Verification items for this drawing (mm, ordinates from the low corner). Coordinates: 2 decimals unless noted, no trailing zeros. Write each loop counter-clockwise with the first axis right and the second up, starting at its lowest first coordinate (ties: lowest second). Pieces come first, ordered by that corner, then holes. Notation, with made-up numbers: M -7,-20.5 L 41,-20.5 A15 cw 41,4.5 Z; hole C 12.5,4.25 d2. An arc over 180 degrees is marked long. Put each result on its own line as item: value. Start each with the question number.
1) Cross-section at C-C on z = 237.5. Record the cut outline in (x, y).
2) Cross-section at A-A on x = 32.5. Record the cut outline in (y, z).
3) Cross-section at D-D on y = 150.5. Record the cut outline in (x, z).
4) Cross-section at B-B on y = 40.5. Record the cut outline in (x, z).
5) Gauge pin test, flat ends, axial feed: pin 1 (8 mm diameter, centred on y = 167.5, z = 715.5, fed in from +X); pin 2 (1.5 mm diameter, centred on y = 124.5, z = 723, fed in from -X). Record the tip position at first contact, or that the pin passes through.
6) Scan lines: line 1 along X through (y, z) = (156, 626); line 2 along Z through (x, y) = (48, 13.5); line 3 along Y through (x, z) = (32.5, 671). Record each from-to range of solid material in increasing order.
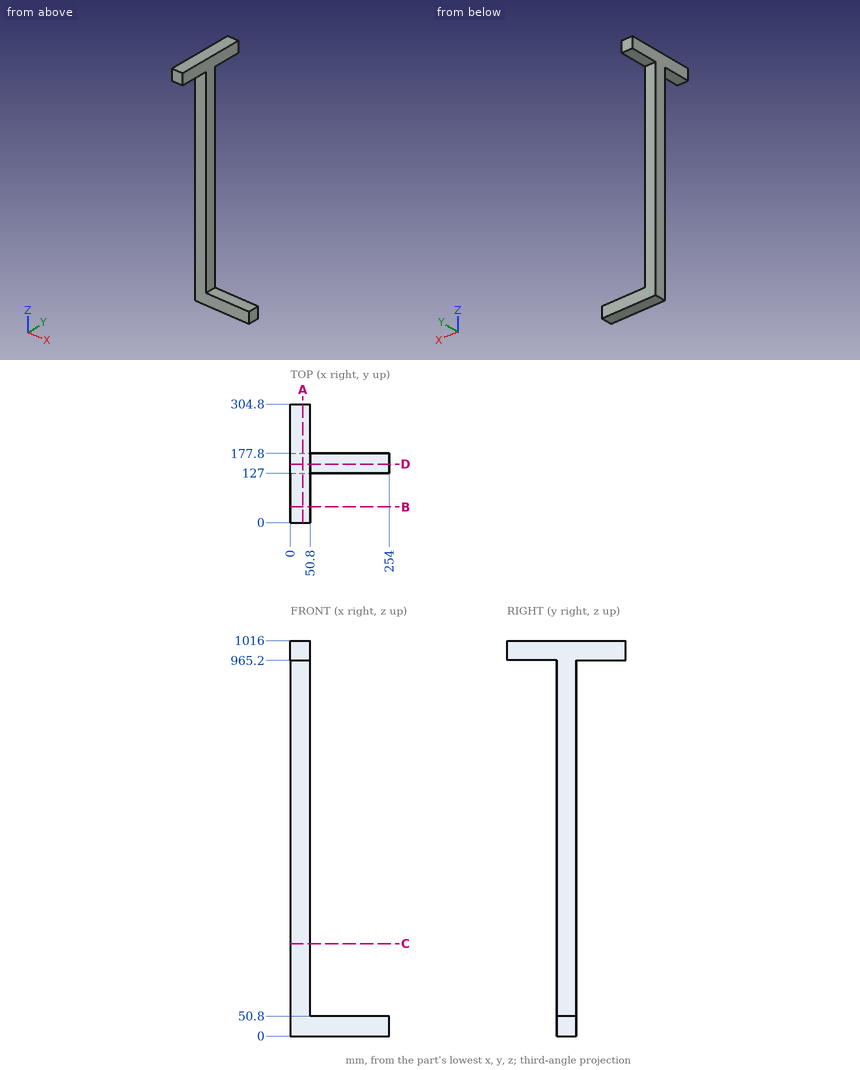
Answer key:
1. outline: M 0,127 L 50.8,127 L 50.8,177.8 L 0,177.8 Z
2. outline: M 0,965.2 L 127,965.2 L 127,0 L 177.8,0 L 177.8,965.2 L 304.8,965.2 L 304.8,1016 L 0,1016 Z
3. outline: M 0,0 L 254,0 L 254,50.8 L 50.8,50.8 L 50.8,1016 L 0,1016 Z
4. outline: M 0,965.2 L 50.8,965.2 L 50.8,1016 L 0,1016 Z
5. pin 1: stops at x = 50.8
5. pin 2: passes through
6. line 1: x = 0 to 50.8
6. line 2: z = 965.2 to 1016
6. line 3: y = 127 to 177.8
